Read the model definition and answer for the solid it produces. Units are mm, in the model's axes. A direction names the side the tool comes from. Give positions to 0.01 mm unless a question says otherwise; leave off trailing zeros. Order: outer loops, then holes, each group sorted by start corner. A loop starts at its lowest first (then second) coordinate and runs counter-clockwise, first axis right, second up. Notation, with made-up numbers: (78.25, 68.5) - (110.25, 68.5) arc R28 ccw to (110.25, 104.5) - close; hole circle Ø11 at (62, 35.25). An arc over 180 degrees is marked (long way). One line per item, written item: value. Start each with the question number.
```python
from build123d import *

# Parameters (mm, degrees)
SKETCH1_R                = 1
BOSS_EXTRUDE1_DEPTH      = 2
BOSS_EXTRUDE2_DEPTH      = 4
BOSS_EXTRUDE2_DEPTH_BACK = 2
SKETCH2_W                = 29
SKETCH2_H                = 5
FILLET1_R                = 5
SKETCH3_W                = 3
SKETCH3_H                = 6
BOSS_EXTRUDE3_DEPTH      = 8
FILLET2_R                = 2
CUT_EXTRUDE1_DEPTH       = 15
CUT_EXTRUDE1_DEPTH_BACK  = 7
SKETCH4_R                = 1.25


with BuildPart() as part:
    # Sketch1 → Boss-Extrude1 (new body)
    with BuildSketch(Plane(origin=(0, 0, 0), x_dir=(1, 0, 0), z_dir=(0, 1, 0))):
        with BuildLine():
            Line((24.9, 26), (25, 26))
            ThreePointArc((25, 26), (27.828427125, 24.828427125), (29, 22))
            Line((29, 22), (29, 0))
            Line((29, 0), (0, 0))
            Line((0, 0), (0, 22))
            ThreePointArc((0, 22), (1.171572875, 24.828427125), (4, 26))
            Line((4, 26), (4.1, 26))
            ThreePointArc((4.1, 26), (6.857716447, 24.857716447), (8, 22.1))
            Line((8, 22.1), (8, 4.5))
            Line((8, 4.5), (21, 4.5))
            Line((21, 4.5), (21, 22.1))
            ThreePointArc((21, 22.1), (22.142283553, 24.857716447), (24.9, 26))
        make_face()
        with Locations(Location((3.95, 22, 0), (0, 0, 270))):
            Circle(SKETCH1_R, mode=Mode.SUBTRACT)
        with Locations(Location((25.05, 22, 0), (0, 0, 270))):
            Circle(SKETCH1_R, mode=Mode.SUBTRACT)
        with Locations(Location((25.05, 9.4, 0), (0, 0, 270))):
            Circle(SKETCH1_R, mode=Mode.SUBTRACT)
        with Locations(Location((3.95, 9.4, 0), (0, 0, 270))):
            Circle(SKETCH1_R, mode=Mode.SUBTRACT)
    extrude(amount=BOSS_EXTRUDE1_DEPTH)

    # Sketch2 → Boss-Extrude2 (add, two sides: drawn at the far end of the back side and taken through both)
    with BuildSketch(Plane(origin=(0, 2, 0), x_dir=(1, 0, 0), z_dir=(0, 1, 0)).offset(-BOSS_EXTRUDE2_DEPTH_BACK)):
        with Locations((14.5, -2.5)):
            Rectangle(SKETCH2_W, SKETCH2_H)
    extrude(amount=BOSS_EXTRUDE2_DEPTH + BOSS_EXTRUDE2_DEPTH_BACK)

    # Fillet1
    # the kernel refuses this fillet: 5 mm, written as the material it adds along each edge
    with BuildSketch(Plane(origin=(29, 2, 0), x_dir=(0, 0, -1), z_dir=(-1, 0, 0))) as fillet1_piece_1_section:
        with BuildLine():
            CenterArc((4.898979486, -5), FILLET1_R, 90, 78.463040967)
            Line((0, -4), (0, 0))
            Line((0, 0), (4.898979486, 0))
        make_face()
    fillet1_piece_1 = extrude(amount=41.247448714, mode=Mode.PRIVATE)
    fillet1_piece_1 = split(fillet1_piece_1, bisect_by=Plane(origin=(21, 2, 0), z_dir=(1, 0, 0)), keep=Keep.TOP, mode=Mode.PRIVATE)
    add(fillet1_piece_1)
    with BuildSketch(Plane(origin=(29, 2, 0), x_dir=(0, 0, -1), z_dir=(-1, 0, 0))) as fillet1_piece_2_section:
        with BuildLine():
            CenterArc((4.898979486, -5), FILLET1_R, 90, 78.463040967)
            Line((0, -4), (0, 0))
            Line((0, 0), (4.898979486, 0))
        make_face()
    fillet1_piece_2 = extrude(amount=29, mode=Mode.PRIVATE)
    fillet1_piece_2 = split(fillet1_piece_2, bisect_by=Plane(origin=(29, 2, -4.5), z_dir=(0, 0, 1)), keep=Keep.TOP, mode=Mode.PRIVATE)
    add(fillet1_piece_2)
    with BuildSketch(Plane(origin=(41.247448714, 2, 0), x_dir=(0, 0, -1), z_dir=(-1, 0, 0))) as fillet1_piece_3_section:
        with BuildLine():
            CenterArc((4.898979486, -5), FILLET1_R, 90, 78.463040967)
            Line((0, -4), (0, 0))
            Line((0, 0), (4.898979486, 0))
        make_face()
    fillet1_piece_3 = extrude(amount=41.247448714, mode=Mode.PRIVATE)
    fillet1_piece_3 = split(fillet1_piece_3, bisect_by=Plane(origin=(8, 2, 0), z_dir=(-1, 0, 0)), keep=Keep.TOP, mode=Mode.PRIVATE)
    add(fillet1_piece_3)

    # Sketch3 → Boss-Extrude3 (add)
    with BuildSketch(Plane.XY.offset(5)):
        with Locations((8, 3)):
            Rectangle(SKETCH3_W, SKETCH3_H)
        with Locations((21, 3)):
            Rectangle(SKETCH3_W, SKETCH3_H)
    extrude(amount=BOSS_EXTRUDE3_DEPTH)

    # Fillet2
    fillet2_edges = [part.edges().sort_by_distance(p)[0] for p in [
        (9.5, 3, 5),
        (6.5, 3, 5),
        (19.5, 3, 5),
        (22.5, 3, 5),
    ]]
    fillet(fillet2_edges, radius=FILLET2_R)

    # Sketch4 → Cut-Extrude1 (cut, two sides: drawn at the far end of the back side and taken through both)
    with BuildSketch(Plane(origin=(9.5, 0, 0), x_dir=(0, 0, -1), z_dir=(1, 0, 0)).offset(-CUT_EXTRUDE1_DEPTH_BACK)):
        with Locations(Location((-10, 3, 0), (0, 0, 180))):
            Circle(SKETCH4_R)
    extrude(amount=CUT_EXTRUDE1_DEPTH + CUT_EXTRUDE1_DEPTH_BACK, mode=Mode.SUBTRACT)


solid = part.part
```
1) Section C-C on x = 20.5 is taken. Write down the section's boundary in (y, z).
2) Each of these flat-tipped pins is pushed along its axis until it touches: pin 1 (4 mm diameter, centred on x = 2.5, z = -18, fed in from +Y); pin 2 (2 mm diameter, centred on x = 1.5, y = 4.5, fed in from +Z); pin 3 (1 mm diameter, centred on x = 13.5, y = 1, fed in from -Z); pin 4 (1.2 mm diameter, centred on x = 3.95, z = -22, fed in from +Y). Where does it stop, or does it pass through?
3) Section A-A on z = -9.4 is taken. Write down the section's boundary in (x, y), plus the area to 3 significant figures.
4) The mould has two halves that part along Z. Classify faces 1 (the cylindrical face through (27.797, 0.986, -24.859)), 2 (the flat face through (14, 6, 4)), 3 (the cylindrical face through (20.98, 2.95, 8.75)): +Z half, -Z half, draft (parallel to the pull), parting line (faces both ways), or undercut.
5) Find the intervals of material crossed by probe 1 along X at (y, z) = (1.2, -22); probe 2 along Y at (x, z) = (7.35, 10); probe 3 along X at (y, z) = (4.5, 10.5), in increasing order. Write a range as from..to.
6) For faces 4 (the cylindrical face through (6.827, 0.986, -24.888)), 5 (the flat face through (9.5, 3, 8.6)), 6 (the flat face through (27, 3, 5)), 7 (the flat face through (2, 3, 5)), determine the directions among +Z, -Z, +X, -X, +Y, -Y from which every point of the face is accessible in a straight line to the end or side of a thin tool.
7) Section D-D on y = 3.75 is taken. Write down the section's boundary in (x, z), plus the area to 3 significant figures.
8) Section B-B on z = -14.5 is taken. Write down the section's boundary in (x, y).
Solved:
1. outline: (0, -4.5) - (2.02, -4.5) arc R5 cw to (6, 0) - (6, 13) - (0, 13) - close; hole circle Ø2.5 at (3, 10)
2. pin 1: stops at y = 2
2. pin 2: stops at z = 5
2. pin 3: stops at z = -4.5
2. pin 4: passes through
3. outline: (0, 0) - (2.95, 0) - (2.95, 2) - (0, 2) - close; (4.95, 0) - (8, 0) - (8, 2) - (4.95, 2) - close; (21, 0) - (24.05, 0) - (24.05, 2) - (21, 2) - close; (26.05, 0) - (29, 0) - (29, 2) - (26.05, 2) - close
3. area: 24.0 mm2
4. face 1: -Z half
4. face 2: draft
4. face 3: undercut
5. probe 1: x = 0..2.95, 4.95..8, 21..24.05, 26.05..29
5. probe 2: y = 0..1.75, 4.25..6
5. probe 3: x = 6.5..9.5, 19.5..22.5
6. face 4: -Z, +Y, -Y
6. face 5: +Z, +Y, -Y
6. face 6: +Z, +X, +Y, -Y
6. face 7: +Z, -X, +Y, -Y
7. outline: (0, -1.1) - (29, -1.1) - (29, 5) - (24.5, 5) arc R2 cw to (22.5, 7) - (22.5, 9) - (19.5, 9) - (19.5, 7) arc R2 cw to (17.5, 5) - (11.5, 5) arc R2 cw to (9.5, 7) - (9.5, 9) - (6.5, 9) - (6.5, 7) arc R2 cw to (4.5, 5) - (0, 5) - close; (6.5, 11) - (9.5, 11) - (9.5, 13) - (6.5, 13) - close; (19.5, 11) - (22.5, 11) - (22.5, 13) - (19.5, 13) - close
7. area: 216 mm2
8. outline: (0, 0) - (8, 0) - (8, 2) - (0, 2) - close; (21, 0) - (29, 0) - (29, 2) - (21, 2) - close
